```python
from build123d import *

# Parameters (mm, degrees)
SKETCH_1_R          = 4
EXTRUDE_1_DEPTH     = 45.2
SKETCH_4_R          = 1.45
CUT_EXTRUDE_3_DEPTH = 8
CUT_EXTRUDE_4_DEPTH = 60


with BuildPart() as part:
    # 草图1 → 凸台-拉伸1 (new body)
    with BuildSketch(Plane.XY):
        Circle(SKETCH_1_R)
    extrude(amount=EXTRUDE_1_DEPTH)

    # 草图4 → 切除-拉伸3 (cut)
    with BuildSketch(Plane(origin=(0, 0, 0), x_dir=(-1, 0, 0), z_dir=(0, 0, -1))):
        Circle(SKETCH_4_R)
    extrude(amount=-CUT_EXTRUDE_3_DEPTH, mode=Mode.SUBTRACT)

    # 草图5 → 切除-拉伸4 (cut)
    with BuildSketch(Plane(origin=(0, 0, 0), x_dir=(-1, 0, 0), z_dir=(0, 0, -1))):
        with BuildLine():
            Line((0, -4), (0, 4))
            ThreePointArc((0, 4), (-4, 0), (0, -4))
        make_face()
    extrude(amount=-CUT_EXTRUDE_4_DEPTH, mode=Mode.SUBTRACT)


solid = part.part
```
Work out the finished part from the listing and answer in its coordinate system (mm). A direction names the side the tool comes from. Coordinates: 2 decimals unless noted, no trailing zeros. Write each loop counter-clockwise with the first axis right and the second up, starting at its lowest first coordinate (ties: lowest second). Pieces come first, ordered by that corner, then holes.
Q1. Each of these flat-tipped pins is pushed along its axis until it touches: pin 1 Ø2 at (y, z) = (2, 23) entering from -X; pin 2 Ø1.2 at (x, y) = (-1, -0.5) entering from -Z. Where does it stop, or does it pass through?
Q2. A cutting plane is placed at B-B, the plane x = -0.55. Give the vertices of the cut face in (y, z), then the cut area to 3 significant figures.
Q3. Which of the six approach directions +Z, -Z, +X, -X, +Y, -Y give full straight-line access (tool end or side, diameter ignored) to faces 1 (the face through (-1, 0, 8)), 2 (the face through (-2, 0, 45.2))?
Q4. A cutting plane is placed at A-A, the plane y = 0. Give the vertices of the cut face in (x, z).
Q5. A cutting plane is placed at C-C, the plane z = 15. Give the vertices of the cut face in (x, y), then the cut area to 3 significant figures.
Q6. A cutting plane is placed at D-D, the plane y = 2.5. Give the vertices of the cut face in (x, z), then the cut area to 3 significant figures.
Q7. Determine the mould class of faces 3 (the face through (0, 0, 22)), 4 (the face through (-4, 0, 22)), 5 (the face through (-1.45, -0.03, 3.94)) for opening direction Y: released by +Y, released by -Y, zero draft, split by the parting line, or undercut.
Q8. Find the intervals of material crossed by line 1 (Y direction, x = -0.2, z = 22) (3 decimals); line 2 (Z direction, x = -0.7, y = -0.5); line 3 (X direction, y = -3, z = 37.5), in increasing order.
Findings below:
1. pin 1: stops at x = -3.87
1. pin 2: stops at z = 0
2. outline: (-3.96, 0) - (-1.34, 0) - (-1.34, 8) - (1.34, 8) - (1.34, 0) - (3.96, 0) - (3.96, 45.2) - (-3.96, 45.2) - close
2. area: 337 mm2
3. face 1: -Z, +X
3. face 2: +Z, +X, -X, +Y, -Y
4. outline: (-4, 0) - (-1.45, 0) - (-1.45, 8) - (0, 8) - (0, 45.2) - (-4, 45.2) - close
5. outline: (0, -4) - (0, 4) arc R4 ccw to start
5. area: 25.1 mm2
6. outline: (-3.12, 0) - (0, 0) - (0, 45.2) - (-3.12, 45.2) - close
6. area: 141 mm2
7. face 3: zero draft
7. face 4: split by the parting line
7. face 5: undercut
8. line 1: y = -3.995 to 3.995
8. line 2: z = 8 to 45.2
8. line 3: x = -2.65 to 0
